Read the model definition and answer for the solid it produces. Units are mm, in the model's axes. Coordinates: 2 decimals unless noted, no trailing zeros. Write each loop counter-clockwise with the first axis right and the second up, starting at its lowest first coordinate (ties: lowest second). Pieces come first, ordered by that corner, then holes. Notation, with made-up numbers: (28.5, 22.5) -> (85.5, 22.5) arc R18 cw to (85.5, 38.5) -> close; hole circle Ø9 at (44, 27.25). An arc over 180 degrees is marked (long way). Write item = value, one per line. Start each with the question number.
1) Section C-C (z = 3.4) is taken. Determine the outline of the cut face in (x, y) (3 decimals), plus the area to 3 significant figures.
2) Find the intervals of material crossed by line 1 along X through (y, z) = (0, 1.75); line 2 along Y through (x, z) = (-120.5, 0.65); line 3 along Y through (x, z) = (-56, 3.25), in increasing order. Write a range as from..to.
3) Section B-B (x = 37.5) is taken. Determine the outline of the cut face in (y, z), plus the area to 3 significant figures.
4) Flat-ended cylindrical pins translate along their axes: pin 1 Ø3 at (x, z) = (-34, 2) entering from -Y; pin 2 Ø2.5 at (x, z) = (156, 3.5) entering from -Y; pin 3 Ø2 at (y, z) = (88, 4.5) entering from -X. Find the tip coordinate at first contact, or state that the pin passes through.
5) For a pull along Y with two mould halves and no side action, classify faces 1 (the face through (-127, 45, 5)), 2 (the face through (-111.725, 71.231, 2.465)), 3 (the face through (-166.99, 57.15, 2.46)) as released by +Y, released by -Y, zero draft, split by the parting line, or undercut.
6) Section A-A (y = 0) is taken. Determine the outline of the cut face in (x, z), plus the area to 3 significant figures.
from build123d import *

# Parameters (mm, degrees)
EXTRUDE_2_DEPTH = 5


with BuildPart() as part:
    # 草图1 → 凸台-拉伸2 (new body)
    with BuildSketch(Plane.XY):
        with BuildLine():
            Line((-170, 50), (-170, -50))
            ThreePointArc((-170, -50), (-167.071067812, -57.071067812), (-160, -60))
            Line((-160, -60), (-143.874945699, -60))
            ThreePointArc((-143.874945699, -60), (-138.57164484, -61.522087521), (-134.882761593, -65.625))
            ThreePointArc((-134.882761593, -65.625), (-79.549512883, -127.168687184), (0, -150))
            ThreePointArc((0, -150), (79.549512883, -127.168687184), (134.882761593, -65.625))
            ThreePointArc((134.882761593, -65.625), (138.57164484, -61.522087521), (143.874945699, -60))
            Line((143.874945699, -60), (160, -60))
            ThreePointArc((160, -60), (167.071067812, -57.071067812), (170, -50))
            Line((170, -50), (170, 50))
            ThreePointArc((170, 50), (167.071067812, 57.071067812), (160, 60))
            Line((160, 60), (143.874945699, 60))
            ThreePointArc((143.874945699, 60), (138.57164484, 61.522087521), (134.882761593, 65.625))
            ThreePointArc((134.882761593, 65.625), (0, 150), (-134.882761593, 65.625))
            ThreePointArc((-134.882761593, 65.625), (-138.57164484, 61.522087521), (-143.874945699, 60))
            Line((-143.874945699, 60), (-160, 60))
            ThreePointArc((-160, 60), (-167.071067812, 57.071067812), (-170, 50))
        make_face()
        with BuildLine():
            ThreePointArc((0, -132.5), (132.5, 0), (0, 132.5))
            ThreePointArc((0, 132.5), (-132.5, 0), (0, -132.5))
        make_face(mode=Mode.SUBTRACT)
    extrude(amount=EXTRUDE_2_DEPTH)


solid = part.part
Answer key:
q1.outline = (-170, -50) arc R10 ccw to (-160, -60) -> (-143.875, -60) arc R10 cw to (-134.883, -65.625) arc R150 ccw to (134.883, -65.625) arc R10 cw to (143.875, -60) -> (160, -60) arc R10 ccw to (170, -50) -> (170, 50) arc R10 ccw to (160, 60) -> (143.875, 60) arc R10 cw to (134.883, 65.625) arc R150 ccw to (-134.883, 65.625) arc R10 cw to (-143.875, 60) -> (-160, 60) arc R10 ccw to (-170, 50) -> close; hole circle Ø265 at (0, 0)
q1.area = 21,300 mm^2
q2.line_1 = -170..-132.5, 132.5..170
q2.line_2 = -89.33..-55.1, 55.1..89.33
q2.line_3 = -139.15..-120.08, 120.08..139.15
q3.outline = (-145.24, 0) -> (-127.08, 0) -> (-127.08, 5) -> (-145.24, 5) -> close; (127.08, 0) -> (145.24, 0) -> (145.24, 5) -> (127.08, 5) -> close
q3.area = 182 mm^2
q4.pin_1 = -146.44
q4.pin_2 = -60
q4.pin_3 = -122.19
q5.face_1 = zero draft
q5.face_2 = undercut
q5.face_3 = released by +Y
q6.outline = (-170, 0) -> (-132.5, 0) -> (-132.5, 5) -> (-170, 5) -> close; (132.5, 0) -> (170, 0) -> (170, 5) -> (132.5, 5) -> close
q6.area = 375 mm^2
